Autodesk Inventor part; units mm, degrees
ref_plane "YZ Plane" through (0, 0, 0) normal (1, 0, 0) x (0, 1, 0)
ref_plane "XZ Plane" through (0, 0, 0) normal (0, 1, 0) x (-1, 0, 0)
ref_plane "XY Plane" through (0, 0, 0) normal (0, 0, 1) x (1, 0, 0)
sketch "Sketch1" plane through (0, 0, 0) normal (0, 1, 0) x (-1, 0, 0)
  line L0 (-8, -16) -> (8, -16)
  line L1 (8, -16) -> (8, 16)
  line L2 (8, 16) -> (-8, 16)
  line L3 (-8, 16) -> (-8, -16)
  line L4 (-8, -16) -> (8, 16) construction
  line L5 (8, -16) -> (-8, 16) construction
  point P0 (0, 0)
  dimension "d0" = 16
  dimension "d1" = 32
extrude "Extrusion1" add sketch "Sketch1" along normal blind 1.6
sketch "Sketch2" plane through (0, 1.6, 0) normal (0, 1, 0) x (1, 0, 0)
  line L0 (3.3525, 2.1899) -> (7.3525, 2.1899)
  line L1 (7.3525, 2.1899) -> (7.3525, -5.8101)
  line L2 (7.3525, -5.8101) -> (3.3525, -5.8101)
  line L3 (3.3525, -5.8101) -> (3.3525, 2.1899)
  point P0 (0, 0)
  dimension "d4" = 4
  dimension "d5" = 8
extrude "Extrusion2" add sketch "Sketch2" along normal blind 8
properties part number "boost-converter" material "ABS Plastic"
Input: part model. Units: mm. Frame: model coordinates. A direction names the side the tool comes from. Round coordinates to 2 decimals unless told otherwise and drop trailing zeros. Write each loop counter-clockwise with the first axis right and the second up, starting at its lowest first coordinate (ties: lowest second). Pieces come first, ordered by that corner, then holes.
1) Cut plane C-C (z = -4). Return the cut outline in (x, y).
2) Ray query, L1, parallel to Y at x = -1, z = -7.5; L2, parallel to Z at x = 6.25, y = 3; L3, parallel to X at y = 6.25, z = 1. Return the intervals inside material, ascending.
3) Cut plane A-A (x = 3.75). Return the cut outline in (y, z), then the cut area to 3 significant figures.
4) Contact query for flat-ended pins moving along their axis: P1, Ø8, axis at x = 4.5, z = -12, coming from the +Y side; P2, Ø4, axis at y = 5, z = 6.5, coming from the +X side; P3, Ø2, axis at x = 6, y = 7, coming from the -Z side. Output: stop coordinate, or through.
5) Reachability of faces 1 (the flat face through (5, 6, -2.19)), 2 (the flat face through (5, 6, 5.81)), 3 (the flat face through (7.352, 6, 2)), 4 (the flat face through (0, 1, -16)), 5 (the flat face through (3.352, 6, 2)) from +Z, -Z, +X, -X, +Y, -Y: full face, straight path, thin tool, end or side. Return the list, or none.
6) Cut plane B-B (y = 5.5). Return the cut outline in (x, z).
Geometry says:
1. outline: (-8, 0) - (8, 0) - (8, 1.6) - (-8, 1.6) - close
2. L1: y = 0 to 1.6
2. L2: z = -2.19 to 5.81
2. L3: x = 3.35 to 7.35
3. outline: (0, -16) - (1.6, -16) - (1.6, -2.19) - (9.6, -2.19) - (9.6, 5.81) - (1.6, 5.81) - (1.6, 16) - (0, 16) - close
3. area: 115 mm2
4. P1: stops at y = 1.6
4. P2: stops at x = 7.35
4. P3: stops at z = -2.19
5. face 1: -Z, +X, -X, +Y
5. face 2: +Z, +X, -X, +Y
5. face 3: +Z, -Z, +X, +Y
5. face 4: -Z, +X, -X, +Y, -Y
5. face 5: +Z, -Z, -X, +Y
6. outline: (3.35, -2.19) - (7.35, -2.19) - (7.35, 5.81) - (3.35, 5.81) - close
